```python
from build123d import *

# Parameters (mm, degrees)
CROQUIS1_W              = 16
CROQUIS1_H              = 14
SALIENTE_EXTRUIR1_DEPTH = 2
CROQUIS2_W              = 3
CROQUIS2_H              = 2.5
SALIENTE_EXTRUIR2_DEPTH = 13
CROQUIS4_W              = 3
CROQUIS4_H              = 2.5
CORTAR_EXTRUIR1_DEPTH   = 1.4
CORTAR_EXTRUIR2_START   = 2.480005
CROQUIS5_R              = 4
CORTAR_EXTRUIR2_DEPTH   = 7.5
CROQUIS7_2_R            = 0.6
CORTAR_EXTRUIR4_DEPTH   = 5
CROQUIS7_R              = 0.6
CORTAR_EXTRUIR3_DEPTH   = 4


with BuildPart() as part:
    # Croquis1 → Saliente-Extruir1 (new body)
    with BuildSketch(Plane(origin=(0, 0, 0), x_dir=(1, 0, 0), z_dir=(0, 1, 0))):
        Rectangle(CROQUIS1_W, CROQUIS1_H)
    extrude(amount=SALIENTE_EXTRUIR1_DEPTH)

    # Croquis2 → Saliente-Extruir2 (add)
    with BuildSketch(Plane(origin=(0, 0, 0), x_dir=(1, 0, 0), z_dir=(0, 1, 0))):
        Polygon((5.890002582, 5.5), (5.890002582, -5.5), (8, -5.5), (8, 7), (-8, 7), (-8, -5.5), (-5.890002582, -5.5), (-5.890002582, 5.5), (-3.409997418, 5.5), (-3.409997418, 3), (-0.409997418, 3), (-0.409997418, 5.5), (1.090002582, 5.5), (1.090002582, 3), (4.090002582, 3), (4.090002582, 5.5), align=None)
        with Locations((-1.909997418, -4.25)):
            Rectangle(CROQUIS2_W, CROQUIS2_H)
        with Locations((2.590002582, -4.25)):
            Rectangle(CROQUIS2_W, CROQUIS2_H)
    extrude(amount=SALIENTE_EXTRUIR2_DEPTH)

    # Croquis4 → Cortar-Extruir1 (cut)
    with BuildSketch(Plane(origin=(0, 13, 0), x_dir=(1, 0, 0), z_dir=(0, 1, 0))):
        with Locations((-1.909997418, -4.25)):
            Rectangle(CROQUIS4_W, CROQUIS4_H)
        with Locations((2.590002582, -4.25)):
            Rectangle(CROQUIS4_W, CROQUIS4_H)
        with Locations((2.590002582, 4.25)):
            Rectangle(CROQUIS4_W, CROQUIS4_H)
        with Locations((-1.909997418, 4.25)):
            Rectangle(CROQUIS4_W, CROQUIS4_H)
    extrude(amount=-CORTAR_EXTRUIR1_DEPTH, mode=Mode.SUBTRACT)

    # Croquis5 → Cortar-Extruir2 (cut)
    with BuildSketch(Plane(origin=(-5.890002582, 0, 0), x_dir=(0, 0, -1), z_dir=(1, 0, 0)).offset(CORTAR_EXTRUIR2_START)):
        with Locations((0, 6.5)):
            Circle(CROQUIS5_R)
    extrude(amount=CORTAR_EXTRUIR2_DEPTH, mode=Mode.SUBTRACT)

    # Croquis7<2> → Cortar-Extruir4 (cut)
    with BuildSketch(Plane(origin=(-5.890002582, 0, 0), x_dir=(0, 0, -1), z_dir=(1, 0, 0))):
        with Locations((0.020682753, 8.25)):
            Circle(CROQUIS7_2_R)
        with BuildLine():
            Line((-0.579317247, 12), (-0.579317247, 13))
            Line((-0.579317247, 13), (0.620682753, 13))
            Line((0.620682753, 13), (0.620682753, 12))
            ThreePointArc((0.620682753, 12), (0.020682753, 11.4), (-0.579317247, 12))
        make_face()
    extrude(amount=-CORTAR_EXTRUIR4_DEPTH, mode=Mode.SUBTRACT)

    # Croquis7 → Cortar-Extruir3 (cut)
    with BuildSketch(Plane(origin=(-5.890002582, 0, 0), x_dir=(0, 0, -1), z_dir=(1, 0, 0))):
        with Locations((0.020682753, 8.25)):
            Circle(CROQUIS7_R)
        with BuildLine():
            Line((-0.579317247, 12), (-0.579317247, 13))
            Line((-0.579317247, 13), (0.620682753, 13))
            Line((0.620682753, 13), (0.620682753, 12))
            ThreePointArc((0.620682753, 12), (0.020682753, 11.4), (-0.579317247, 12))
        make_face()
    extrude(amount=-CORTAR_EXTRUIR3_DEPTH, mode=Mode.SUBTRACT)


solid = part.part
```
Could you check a few things on this model? Use its own coordinates, in mm. A direction names the side the tool comes from. Round coordinates to 2 decimals unless told otherwise and drop trailing zeros. Loops run counter-clockwise (first coordinate to the right, second up) from the corner with the lowest first, then second, coordinate; pieces in that order, holes last. Notation, with made-up numbers: (14.5, 56.25) - (69.5, 56.25) arc R9 cw to (69.5, 72.25) - close; hole circle Ø2 at (8.25, 34). An arc over 180 degrees is marked (long way). Answer as CSV lines item,"result".
1. On a 3-axis mill with a long thin cutter (end or side, diameter ignored), from which of +Z, -Z, +X, -X, +Y, -Y can I reach the whole of each face in a straight line? I mean faces 4 (the face through (-6.93, 7.664, 0.109)), 5 (the face through (-2, 10, -3)), 6 (the face through (-1.9, 6.5, 4)), 7 (the face through (-6.9, 12.5, -0.621)). Say none if no direction works.
Filled in:
face 4,"-X"
face 5,"+Y"
face 6,"none"
face 7,"-X, +Y"
2. I want a section at D-D on z = -3.75. List the corners of the cut face in (x, y) for me.
Filled in:
outline,"(-8, 0) - (8, 0) - (8, 13) - (5.89, 13) - (5.89, 2) - (4.09, 2) - (4.09, 5.11) - (1.09, 5.11) - (1.09, 2) - (-0.41, 2) - (-0.41, 5.11) - (-3.41, 5.11) - (-3.41, 2) - (-5.89, 2) - (-5.89, 13) - (-8, 13) - close; (-3.41, 7.89) - (-0.41, 7.89) - (-0.41, 11.6) - (-3.41, 11.6) - close; (1.09, 7.89) - (4.09, 7.89) - (4.09, 11.6) - (1.09, 11.6) - close"
3. We'd pull the mould along Y, two halves only. Please class faces 1 (the face through (4.09, 7, -5)), 2 (the face through (2.6, 6.5, 4)), 3 (the face through (2, 13, -6)): +Y half, -Y half, draft (parallel to the pull), parting line (faces both ways), or undercut.
Filled in:
face 1,"draft"
face 2,"undercut"
face 3,"+Y half"
4. Please list where these lines run through material, in increasing order: line 1 along X through (y, z) = (3.25, -5); line 2 along X through (y, z) = (4.5, -2.5); line 3 along Z through (x, y) = (-6.75, 3.25). Write a range as [from, to].
Filled in:
line 1,"x = [-8, -5.89], [-3.41, -0.41], [1.09, 4.09], [5.89, 8]"
line 2,"x = [-8, -5.89], [5.89, 8]"
line 3,"z = [-7, 5.5]"
5. For pin 1 Ø4 at (x, z) = (0, 2.5) entering from +Y; pin 2 Ø3 at (x, y) = (-4.5, 8.5) entering from +Z; pin 3 Ø2 at (x, y) = (-4.5, 11) entering from +Z, each with a flat end and sliding along its axis, tell me the tip position at first contact or that it passes through.
Filled in:
pin 1,"stops at y = 11.6"
pin 2,"stops at z = 5.5"
pin 3,"stops at z = -5.5"
6. I want a section at A-A on y = 3. List the corners of the cut face in (x, z) for me, then the cut area to 3 significant figures.
Filled in:
outline,"(-8, -7) - (8, -7) - (8, 5.5) - (5.89, 5.5) - (5.89, -5.5) - (4.09, -5.5) - (4.09, -3) - (1.09, -3) - (1.09, -5.5) - (-0.41, -5.5) - (-0.41, -3) - (-3.41, -3) - (-3.41, -5.5) - (-5.89, -5.5) - (-5.89, 5.5) - (-8, 5.5) - close; (-3.41, 3) - (-0.41, 3) - (-0.41, 5.5) - (-3.41, 5.5) - close; (1.09, 3) - (4.09, 3) - (4.09, 5.5) - (1.09, 5.5) - close"
area,"100 mm^2"
7. I want a section at C-C on y = 8.25. List the corners of the cut face in (x, z) for me.
Filled in:
outline,"(-8, -7) - (8, -7) - (8, 5.5) - (5.89, 5.5) - (5.89, -5.5) - (4.09, -5.5) - (4.09, -3.6) - (1.09, -3.6) - (1.09, -5.5) - (-0.41, -5.5) - (-0.41, -3.6) - (-3.41, -3.6) - (-3.41, -5.5) - (-5.89, -5.5) - (-5.89, -0.62) - (-8, -0.62) - close; (-8, 0.58) - (-5.89, 0.58) - (-5.89, 5.5) - (-8, 5.5) - close; (-3.41, 3.6) - (-0.41, 3.6) - (-0.41, 5.5) - (-3.41, 5.5) - close; (1.09, 3.6) - (4.09, 3.6) - (4.09, 5.5) - (1.09, 5.5) - close"
8. I want a section at B-B on x = -2. List the corners of the cut face in (y, z) for me, then the cut area to 3 significant figures.
Filled in:
outline,"(0, -7) - (13, -7) - (13, -5.5) - (11.6, -5.5) - (11.6, -3) - (9.15, -3) arc R4 cw to (3.85, -3) - (2, -3) - (2, 3) - (3.85, 3) arc R4 cw to (9.15, 3) - (11.6, 3) - (11.6, 5.5) - (2, 5.5) - (2, 7) - (0, 7) - close"
area,"85.2 mm^2"
